Autodesk Inventor part; units mm, degrees
ref_plane "YZ Plane" through (0, 0, 0) normal (1, 0, 0) x (0, 1, 0)
ref_plane "XZ Plane" through (0, 0, 0) normal (0, 1, 0) x (-1, 0, 0)
ref_plane "XY Plane" through (0, 0, 0) normal (0, 0, 1) x (1, 0, 0)
sketch "Esboço1" plane through (0, 0, 0) normal (0, 0, 1) x (1, 0, 0)
  circle A0 centre (0, 0) radius 20
  circle A1 centre (0, 0) radius 24
  dimension "d0" = 40
  dimension "d1" = 48
extrude "Extrusão1" add sketch "Esboço1" along normal mid plane 30.65
chamfer "Chanfro1" distance 0.5 angle 45 2 edges at (-24, 0, 15.325) (-24, 0, -15.325)
Can you work these out from the model? Positions are in its coordinate system, mm. Coordinates: 2 decimals unless noted, no trailing zeros. Write each loop counter-clockwise with the first axis right and the second up, starting at its lowest first coordinate (ties: lowest second). Pieces come first, ordered by that corner, then holes. Notation, with made-up numbers: (-23.75, 42.25) -> (18.25, 42.25) arc R26 ccw to (18.25, 58.25) -> close; hole circle Ø10 at (-33.75, 17). An arc over 180 degrees is marked (long way). Write each question's results on one line, items separated by ' | '. Start each with the question number.
Q1. If I drill on probe 1 along X at (y, z) = (0.5, -9); probe 2 along Y at (x, z) = (0, 4); probe 3 along X at (y, z) = (-10.5, 5), over which ranges is the centre line in solid material (lowest first)?
Q2. Imagine slicing it at A-A (y = 0). Write out the boundary of the cut face in (x, z) (3 decimals), then the cut area to 3 significant figures.
Q3. We'd pull the mould along X, two halves only. Please class faces 1 (the face through (-4.336, -19.524, 0.215)), 2 (the face through (-23.977, -1.055, -0.208)), 3 (the face through (7, 19, 15.325)): +X half, -X half, draft (parallel to the pull), parting line (faces both ways), or undercut.
Q4. I'm going to push flat-ended pins straight in: pin 1 (1 mm diameter, centred on x = 13.5, z = 9.5, fed in from +Y); pin 2 (3 mm diameter, centred on y = -12.5, z = 7.5, fed in from +X); pin 3 (3 mm diameter, centred on y = 4.5, z = -10.5, fed in from +X). Where does each tip first touch, or does it pass through?
Q5. Imagine slicing it at C-C (z = 11.5). Write out the boundary of the cut face in (x, y), then the cut area to 3 significant figures.
Taken from the geometry:
1) probe 1: x = -23.99 to -19.99, 19.99 to 23.99 | probe 2: y = -24 to -20, 20 to 24 | probe 3: x = -21.58 to -17.02, 17.02 to 21.58
2) outline: (-24, -14.825) -> (-23.5, -15.325) -> (-20, -15.325) -> (-20, 15.325) -> (-23.5, 15.325) -> (-24, 14.825) -> close; (20, -15.325) -> (23.5, -15.325) -> (24, -14.825) -> (24, 14.825) -> (23.5, 15.325) -> (20, 15.325) -> close | area: 245 mm^2
3) face 1: undercut | face 2: parting line | face 3: draft
4) pin 1: stops at y = 20.17 | pin 2: stops at x = 21.33 | pin 3: stops at x = 23.81
5) outline: circle Ø48 at (0, 0); hole circle Ø40 at (0, 0) | area: 553 mm^2
